Work out the finished part from the listing and answer in its coordinate system (mm). A direction names the side the tool comes from. Give positions to 0.01 mm unless a question says otherwise; leave off trailing zeros. Order: outer loops, then holes, each group sorted by start corner. A loop starts at its lowest first (then second) coordinate and runs counter-clockwise, first axis right, second up.
```python
from build123d import *

# Parameters (mm, degrees)
ESQUISSE1_W        = 12.8
ESQUISSE1_H        = 9
BOSS_EXTRU_1_DEPTH = 3.5
BOSS_EXTRU_2_DEPTH = 1
ESQUISSE3_R        = 3.1
BOSS_EXTRU_3_DEPTH = 8


with BuildPart() as part:
    # Esquisse1 → Boss.-Extru.1 (new, symmetric)
    with BuildSketch(Plane.XY):
        with Locations((0, -4.5)):
            Rectangle(ESQUISSE1_W, ESQUISSE1_H)
    extrude(amount=BOSS_EXTRU_1_DEPTH, both=True)

    # Esquisse2 → Boss.-Extru.2 (add)
    with BuildSketch(Plane(origin=(0, 0, 0), x_dir=(1, 0, 0), z_dir=(0, 1, 0))):
        with BuildLine():
            Line((1.936491673, 3.5), (-1.936491673, 3.5))
            ThreePointArc((-1.936491673, 3.5), (-4, 0), (-1.936491673, -3.5))
            Line((-1.936491673, -3.5), (1.936491673, -3.5))
            ThreePointArc((1.936491673, -3.5), (4, 0), (1.936491673, 3.5))
        make_face()
    extrude(amount=BOSS_EXTRU_2_DEPTH)

    # Esquisse3 → Boss.-Extru.3 (add)
    with BuildSketch(Plane(origin=(0, 1, 0), x_dir=(1, 0, 0), z_dir=(0, 1, 0))):
        with Locations(Location((0, 0, 0), (0, 0, 180))):
            Circle(ESQUISSE3_R)
    extrude(amount=BOSS_EXTRU_3_DEPTH)

    # Lissage1: read off the stored shape, not the designer's step
    # Lissage1: loft between two sections, ruled curve by curve
    lissage1_from = [
        Edge.make_bspline([(-1.5, 21, -0.999999999), (-1.5, 21, -1.18566879), (-1.430190912, 21, -1.564549941), (-1.108880999, 21, -2.068285581), (-0.606403504, 21, -2.416848616), (0, 21, -2.541699349), (0.606403504, 21, -2.416848616), (1.108880999, 21, -2.068285581), (1.430190912, 21, -1.564549941), (1.5, 21, -1.18566879), (1.5, 21, -0.811971834), (1.5, 21, -0.473320268), (1.5, 21, 0), (1.5, 21, 0.473320268), (1.5, 21, 0.811971834), (1.5, 21, 1.18566879), (1.430190912, 21, 1.564549941), (1.108880999, 21, 2.068285581), (0.606403504, 21, 2.416848616), (0, 21, 2.541699349), (-0.606403504, 21, 2.416848616), (-1.108880999, 21, 2.068285581), (-1.430190912, 21, 1.564549941), (-1.5, 21, 1.18566879), (-1.5, 21, 0.811971834), (-1.5, 21, 0.473320268), (-1.5, 21, 0), (-1.5, 21, -0.473320268), (-1.5, 21, -0.811971834), (-1.5, 21, -0.999999999)], [0, 0, 0, 0, 0.041490919, 0.082981838, 0.124472757, 0.165963676, 0.207454595, 0.248945514, 0.290436432, 0.331927351, 0.331927351, 0.373945514, 0.415963676, 0.457981838, 0.5, 0.5, 0.541490919, 0.582981838, 0.624472757, 0.665963676, 0.707454595, 0.748945514, 0.790436432, 0.831927351, 0.831927351, 0.873945514, 0.915963676, 0.957981838, 1, 1, 1, 1], 3),
    ]
    lissage1_to = [
        Edge.make_bspline([(-1.248075441, 9, -0.832050294), (-1.175771622, 9, -0.940506024), (-1.006710877, 9, -1.133071374), (-0.699452785, 9, -1.34380864), (-0.358220052, 9, -1.471362722), (0, 9, -1.514343967), (0.358220052, 9, -1.471362722), (0.699452785, 9, -1.34380864), (1.006710877, 9, -1.133071374), (1.175771622, 9, -0.940506024), (1.321298058, 9, -0.72221637), (1.449339658, 9, -0.467018972), (1.525563306, 9, 0), (1.449339658, 9, 0.467018972), (1.321298058, 9, 0.72221637), (1.175771622, 9, 0.940506024), (1.006710877, 9, 1.133071374), (0.699452785, 9, 1.34380864), (0.358220052, 9, 1.471362722), (0, 9, 1.514343967), (-0.358220052, 9, 1.471362722), (-0.699452785, 9, 1.34380864), (-1.006710877, 9, 1.133071374), (-1.175771622, 9, 0.940506024), (-1.321298058, 9, 0.72221637), (-1.449339658, 9, 0.467018972), (-1.525563306, 9, 0), (-1.449339658, 9, -0.467018972), (-1.321298058, 9, -0.72221637), (-1.248075441, 9, -0.832050294)], [0, 0, 0, 0, 0.041490919, 0.082981838, 0.124472757, 0.165963676, 0.207454595, 0.248945514, 0.290436432, 0.331927351, 0.331927351, 0.373945514, 0.415963676, 0.457981838, 0.5, 0.5, 0.541490919, 0.582981838, 0.624472757, 0.665963676, 0.707454595, 0.748945514, 0.790436432, 0.831927351, 0.831927351, 0.873945514, 0.915963676, 0.957981838, 1, 1, 1, 1], 3),
    ]
    lissage1 = Solid(Shell([*[Face.make_surface_from_curves(lissage1_from[k], lissage1_to[k]) for k in range(1)], Face(Wire(lissage1_from)), Face(Wire(lissage1_to))]))
    add(lissage1)


solid = part.part
```
1. Straight lines are drawn through the part: probe 1 along Y at (x, z) = (-2, -1.75); probe 2 along Y at (x, z) = (5.25, 1); probe 3 along Z at (x, y) = (-1.25, 16.5). For each, find the intervals that lie inside material, in ascending order.
Findings below:
probe 1: y = -9 to 9
probe 2: y = -9 to 0
probe 3: z = -1.38 to 1.38
2. The part is cut by section A-A (y = 2). Write down the section's boundary in (x, z).
Findings below:
outline: circle Ø6.2 at (0, 0)
3. Which of the six approach directions +Z, -Z, +X, -X, +Y, -Y give full straight-line access (tool end or side, diameter ignored) to faces 1 (the face through (6.4, -5, 0)), 2 (the face through (-2.957, 4.944, 0.931)), 3 (the face through (-4, 0.5, -0.1)), 4 (the face through (0, 21, 0)), 5 (the face through (4, 0.5, 0.1))?
Findings below:
face 1: +Z, -Z, +X, +Y, -Y
face 2: +Y
face 3: -X, +Y
face 4: +Z, -Z, +X, -X, +Y
face 5: +X, +Y
4. Given P1, Ø1, axis at y = 13, z = -2, coming from the -X side; P2, Ø3.5, axis at x = 4, z = 1.5, coming from the +Y side; P3, Ø1, axis at x = -2.5, y = 3.5, coming from the +Z side, each flat-ended and moving along its own axis, determine where each tip first touches the part or whether it passes through.
Findings below:
P1: stops at x = -0.91
P2: stops at y = 9
P3: stops at z = 2.37
